from build123d import *

# Parameters (mm, degrees)
SKETCH1_R           = 3.175
EXTRUDE1_DEPTH      = 31.75
SKETCH2_R           = 1.25
EXTRUDE2_DEPTH      = 5
CHAMFER1_SIZE       = 0.254
EXTRUDE3_DEPTH      = 4.175
EXTRUDE3_DEPTH_BACK = 4.175
SKETCH4_R           = 2.159
SKETCH4_R_2         = 0.254
EXTRUDE4_DEPTH      = 0.0254


with BuildPart() as part:
    # Sketch1 → Extrude1 (new body)
    with BuildSketch(Plane.XY):
        Circle(SKETCH1_R)
    extrude(amount=EXTRUDE1_DEPTH)

    # Sketch2 → Extrude2 (add)
    with BuildSketch(Plane(origin=(0, 0, 0), x_dir=(-1, 0, 0), z_dir=(0, 0, -1))):
        with Locations(Location((0, 0, 0), (0, 0, 180))):  # turned: the seam where the file's is
            Circle(SKETCH2_R)
    extrude(amount=EXTRUDE2_DEPTH)

    # Chamfer1
    chamfer1_edges = [part.edges().sort_by_distance(p)[0] for p in [
        (-1.25, 0, -5),
    ]]
    chamfer(chamfer1_edges, length=CHAMFER1_SIZE)

    # Sketch3 → Extrude3 (cut, two sides)
    with BuildSketch(Plane(origin=(0, 0, 0), x_dir=(0, 0, -1), z_dir=(1, 0, 0))) as extrude3_sk:
        Polygon((-31.75, 0), (-9.525, 0), (-6.35, 3.175), (-31.75, 3.175), align=None)
    extrude(amount=EXTRUDE3_DEPTH, mode=Mode.SUBTRACT)
    extrude(extrude3_sk.sketch, amount=-EXTRUDE3_DEPTH_BACK, mode=Mode.SUBTRACT)

    # Sketch4 → Extrude4 (cut)
    with BuildSketch(Plane(origin=(0, 0, 0), x_dir=(1, 0, 0), z_dir=(0, 1, 0))):
        with Locations(Location((0, -25.4, 0), (0, 0, 270))):  # turned: the seam where the file's is
            Circle(SKETCH4_R)
        with Locations(Location((0, -25.4, 0), (0, 0, 270))):  # turned: the seam where the file's is
            Circle(SKETCH4_R_2, mode=Mode.SUBTRACT)
    extrude(amount=-EXTRUDE4_DEPTH, mode=Mode.SUBTRACT)


solid = part.part
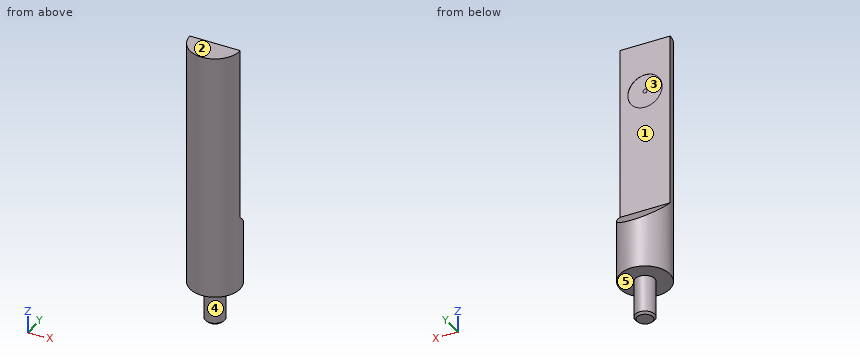
The listing builds one solid part. Answer for the finished solid, in the listing's coordinates (mm). Face numbers are marked on the shaded views. A direction names the side the tool comes from. Coordinates: 2 decimals unless noted, no trailing zeros. Write each loop counter-clockwise with the first axis right and the second up, starting at its lowest first coordinate (ties: lowest second). Pieces come first, ordered by that corner, then holes. Notation, with made-up numbers: (-4.75, 40.5) -> (3.25, 40.5) arc R16 cw to (3.25, 65.5) -> close; hole circle Ø9 at (12.25, 52.5). An arc over 180 degrees is marked (long way). One line per question, with ' | ' between items.
1. Section C-C (y = -2.5) is taken. Determine the outline of the cut face in (x, z), and give its area (3 significant figures).
Verdict:
outline: (-1.96, 0) -> (1.96, 0) -> (1.96, 31.75) -> (-1.96, 31.75) -> close | area: 124 mm^2
2. Given pin 1 Ø1.5 at (x, y) = (2.5, 1.5) entering from -Z; pin 2 Ø1 at (x, z) = (2.5, 3) entering from -Y; pin 3 Ø2 at (x, z) = (0.5, 24.5) entering from +Y, each flat-ended and moving along its own axis, determine where each tip first touches the part or whether it passes through.
Verdict:
pin 1: stops at z = 0 | pin 2: stops at y = -2.47 | pin 3: stops at y = 0
3. Which of the six approach directions +Z, -Z, +X, -X, +Y, -Y give full straight-line access (tool end or side, diameter ignored) to the marked faces 1 and 2?
Verdict:
face 1: +Z, +X, -X, +Y | face 2: +Z, +X, -X, +Y, -Y
4. Straight lines are drawn through the part: line 1 (Y direction, x = 0, z = 13.5) (3 decimals); line 2 (Z direction, x = -1, y = -2.5); line 3 (Y direction, x = 0.5, z = -2.5). For each, find the intervals that lie inside material, in ascending order.
Verdict:
line 1: y = -3.175 to 0 | line 2: z = 0 to 31.75 | line 3: y = -1.15 to 1.15
5. Section A-A (z = 24) is taken. Determine the outline of the cut face in (x, y) (3 decimals).
Verdict:
outline: (-3.175, 0) arc R3.175 ccw to (3.175, 0) -> (1.644, 0) -> (1.644, -0.025) -> (-1.644, -0.025) -> (-1.644, 0) -> close
6. Section B-B (x = -2.5) is taken. Determine the outline of the cut face in (y, z) (3 decimals), and give its area (3 significant figures).
Verdict:
outline: (-1.957, 0) -> (1.957, 0) -> (1.957, 7.568) -> (0, 9.525) -> (0, 31.75) -> (-1.957, 31.75) -> close | area: 78.9 mm^2
7. For a pull along Z with two mould halves and no side action, classify the marked faces 3, 4 and 5 as released by +Z, released by -Z, zero draft, split by the parting line, or undercut.
Verdict:
face 3: undercut | face 4: zero draft | face 5: released by -Z
8. Section D-D (z = 14.5) is taken. Determine the outline of the cut face in (x, y) (3 decimals), and give its area (3 significant figures).
Verdict:
outline: (-3.175, 0) arc R3.175 ccw to (3.175, 0) -> close | area: 15.8 mm^2
